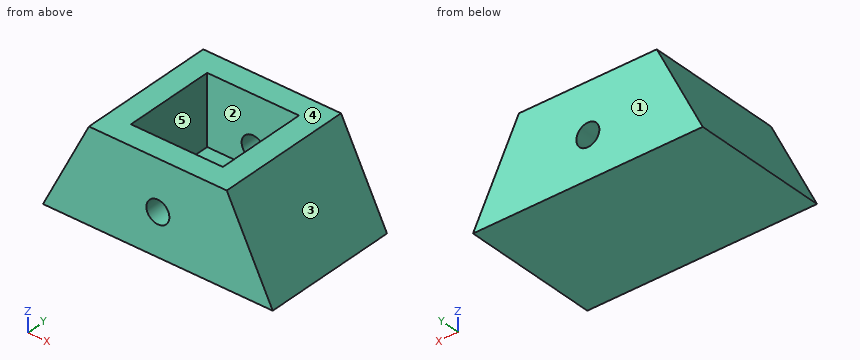
Autodesk Inventor part; units mm, degrees
ref_plane "YZ Plane" through (0, 0, 0) normal (1, 0, 0) x (0, 1, 0)
ref_plane "XZ Plane" through (0, 0, 0) normal (0, 1, 0) x (-1, 0, 0)
ref_plane "XY Plane" through (0, 0, 0) normal (0, 0, 1) x (1, 0, 0)
sketch "Sketch1" plane through (0, 0, 0) normal (0, 0, 1) x (1, 0, 0)
  line L0 (0, 0) -> (30, 0)
  line L1 (30, 0) -> (30, -30)
  line L2 (30, -30) -> (0, -30)
  line L3 (0, -30) -> (0, 0)
  line L4 (0, 0) -> (5, 0)
  line L5 (5, -5.8022) -> (25, -5.8022)
  line L6 (25, -5.8022) -> (25, -25.8022)
  line L7 (25, -25.8022) -> (5, -25.8022)
  line L8 (5, -25.8022) -> (5, -5.8022)
  dimension "d0" = 30
  dimension "d1" = 30
  dimension "d6" = 20
  dimension "d7" = 20
extrude "Extrusion1" add sketch "Sketch1" along normal blind 20 contours L0 L1 L2 L3 | L5 L6 L7 L8
sketch "Sketch2" plane through (0, 0, 20) normal (0, 0, 1) x (1, 0, 0)
  line L0 (30, 0) -> (0, 0)
  line L1 (0, 0) -> (5, 0)
  line L2 (5, -5) -> (25, -5)
  line L3 (25, -5) -> (25, -25)
  line L4 (25, -25) -> (5, -25)
  line L5 (5, -25) -> (5, -5)
  dimension "d8" = 5
extrude "Extrusion2" cut sketch "Sketch2" against normal blind 15
sketch "Sketch3" plane through (0, -30, 0) normal (0, -1, 0) x (1, 0, 0)
  line L0 (0, 0) -> (-10, 0)
  line L1 (0, 0) -> (0, 20)
  line L2 (-10, 0) -> (0, 20)
  dimension "d14" = 10
extrude "Extrusion3" add sketch "Sketch3" against normal blind 30
sketch "Sketch4" plane through (30, -30, 0) normal (0, -1, 0) x (1, 0, 0)
  line L0 (-40, 0) -> (0, 0)
  line L1 (0, 0) -> (10, 0)
  line L2 (0, 0) -> (0, 20)
  line L3 (10, 0) -> (0, 20)
  point P0 (-30, 0)
  dimension "d17" = 10
extrude "Extrusion4" add sketch "Sketch4" against normal blind 30
sketch "Sketch5" plane through (-10, -30, 0) normal (0, -1, 0) x (1, 0, 0)
  line L0 (10, 9.1728) -> (40, 9.1728)
  line L1 (15, 20) -> (35, 20)
  line L2 (25, 20) -> (25, 9.1728)
  circle A0 centre (25, 9.1728) radius 2.5
  point P0 (10, 0)
  dimension "d21" = 5
extrude "Extrusion5" cut sketch "Sketch5" against normal blind 30
equation "\"BendRadius\" = Thickness"
equation "\"BendReliefWidth\" = Thickness"
equation "\"BendReliefDepth\" = 0.5 * Thickness"
equation "\"CornerReliefSize\" = 4 * Thickness"
equation "\"MinimumRemnant\" = 2 * Thickness"
equation "\"TransitionRadius\" = BendRadius"
equation "\"JacobiRadiusSize\" = BendRadius"
equation "\"GapSize\" = Thickness"
properties part number "base de soporte"
The model under review builds one solid part; all positions refer to its coordinate system, in mm. Face numbers are marked on the shaded views. A direction names the side the tool comes from. Coordinates: 2 decimals unless noted, no trailing zeros. Write each loop counter-clockwise with the first axis right and the second up, starting at its lowest first coordinate (ties: lowest second). Pieces come first, ordered by that corner, then holes. Notation, with made-up numbers: (67, 77.25) - (100, 77.25) arc R7 cw to (100, 84.25) - close; hole circle Ø3 at (63.25, 48.25). An arc over 180 degrees is marked (long way). Answer as a JSON object with one key per item and string values. Group by question number.
1. Add section B-B (x = 15). Give the boundary of the cut face in (y, z).
2. Add section D-D (z = 17.5). Give the boundary of the cut face in (x, y).
3. Add section A-A (z = 5.5). Give the boundary of the cut face in (x, y).
4. Machinability: for the marked faces 4 and 5, which of the approach directions +Z, -Z, +X, -X, +Y, -Y give a long, thin tool a straight path to every point of the face, cutting with its end or side? Answer none if there is none.
5. Add section C-C (y = -20.25). Give the boundary of the cut face in (x, z), plus the area to 3 significant figures.
6. Clearance check with flat-ended pins moving along their axes: pin 1 Ø1 at (y, z) = (-7, 4.5) entering from +X; pin 2 Ø12 at (y, z) = (-10, 10.5) entering from +X; pin 3 Ø3 at (x, z) = (15, 9.17) entering from +Y; pin 4 Ø5 at (y, z) = (-6, 16.5) entering from +X. State where each tip first meets the part, or that it passes through.
7. To check wall thickness, follow probe 1 along Z at (x, y) = (15, -1.5); probe 2 along Y at (x, z) = (20, 9); probe 3 along X at (y, z) = (-19.5, 19.25) (3 decimals). State the ranges of each line that lie inside material, in increasing order.
8. Mouldability with a two-part tool opening along X and no side actions: class the marked faces 1, 2 and 3 as pulls with the +X half, pulls with the -X half, needs draft (parallel to the pull), parting line crosses it, or undercut.
Findings:
{
 "1": {"outline": "(-30, 0) - (0, 0) - (0, 6.67) - (-5, 6.67) - (-5, 5) - (-25, 5) - (-25, 6.67) - (-30, 6.67) - close; (-30, 11.67) - (-25, 11.67) - (-25, 20) - (-30, 20) - close; (-5, 11.67) - (0, 11.67) - (0, 20) - (-5, 20) - close"},
 "2": {"outline": "(-1.25, -30) - (31.25, -30) - (31.25, 0) - (-1.25, 0) - close; hole (5, -25) - (25, -25) - (25, -5) - (5, -5) - close"},
 "3": {"outline": "(-7.25, -30) - (37.25, -30) - (37.25, 0) - (-7.25, 0) - close; hole (5, -25) - (25, -25) - (25, -5) - (5, -5) - close"},
 "4": {"face 4": "+Z, +X, -X, +Y, -Y", "face 5": "+Z"},
 "5": {"outline": "(-10, 0) - (40, 0) - (30, 20) - (25, 20) - (25, 5) - (5, 5) - (5, 20) - (0, 20) - close", "area": "500 mm²"},
 "6": {"pin 1": "x = 38", "pin 2": "x = 37.75", "pin 3": "through", "pin 4": "x = 33"},
 "7": {"probe 1": "0 to 6.67, 11.67 to 20", "probe 2": "-30 to -25, -5 to 0", "probe 3": "-0.375 to 5, 25 to 30.375"},
 "8": {"face 1": "needs draft", "face 2": "undercut", "face 3": "pulls with the +X half"}
}
